Check sheet for the drawn part. Datum: minimum x, y, z corner. Units: mm. A direction names the side the tool comes from. Round coordinates to 2 decimals unless told otherwise and drop trailing zeros. Write each loop counter-clockwise with the first axis right and the second up, starting at its lowest first coordinate (ties: lowest second). Pieces come first, ordered by that corner, then holes. Notation, with made-up numbers: M 21.25,51 L 47.25,51 A10 ccw 47.25,64 Z; hole C 22.25,2.5 d2. An arc over 180 degrees is marked long. Answer in a Markdown table with one row per item. Add a question column.
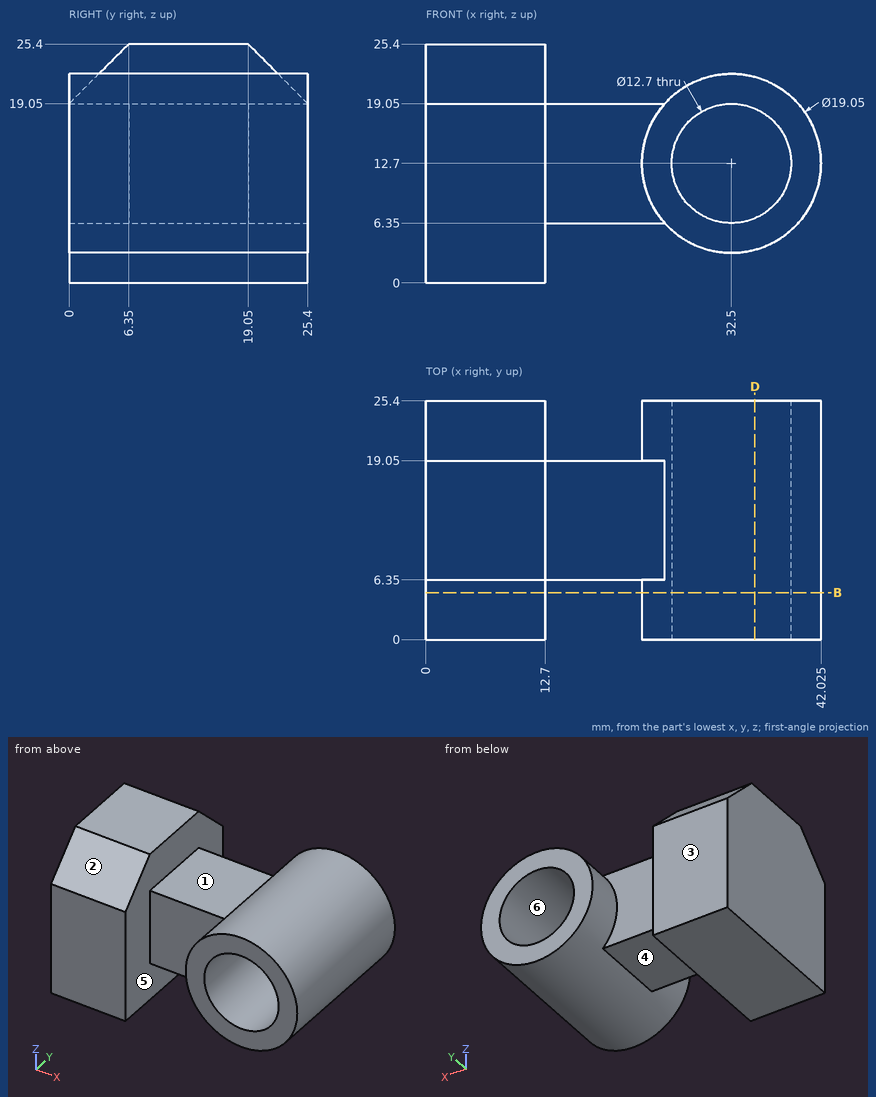
Item 1: Scan lines: probe 1 along X at (y, z) = (22.5, 9) (1 decimal); probe 2 along X at (y, z) = (21.25, 10.25) (1 decimal); probe 3 along Z at (x, y) = (36, 21.75). Record each from-to range of solid material in increasing order. Write a range as from..to.
Item 2: Section check B-B, the plane y = 5. Give the number of separate pieces and of enclosed holes in the cut face, and give its area (3 significant figures).
Item 3: Gauge pin test, flat ends, axial feed: pin 1 Ø7.5 at (y, z) = (7, 14.5) entering from +X (1 decimal); pin 2 Ø5 at (x, y) = (27, 13.5) entering from +Z; pin 3 Ø10 at (x, y) = (21.5, 12) entering from +Z; pin 4 Ø3 at (y, z) = (14.5, 17.5) entering from +X (1 decimal). Record the tip position at first contact, or that the pin passes through.
Item 4: Mould release check, pull along Z, two halves, no side actions. Record for the marked faces 4, 5 and 6: +Z half, -Z half, draft (parallel to the pull), parting line (faces both ways), or undercut.
Item 5: Section check D-D, the plane x = 35. Record the boundary of the cut face in (y, z).
Item 6: Access from +Z, -Z, +X, -X, +Y, -Y to the whole of each face (thin tool, end or side, straight path). Record for the marked faces 1, 2 and 3.
Result sheet:
| question | item | result |
|---|---|---|
| 1 | probe 1 | x = 0..12.7, 23.7..27.3, 37.7..41.3 |
| 1 | probe 2 | x = 0..12.7, 23.3..26.6, 38.4..41.7 |
| 1 | probe 3 | z = 3.84..7.4, 18..21.56 |
| 2 | separate pieces | 2 |
| 2 | enclosed holes | 1 |
| 2 | area | 464 mm^2 |
| 3 | pin 1 | stops at x = 42 |
| 3 | pin 2 | stops at z = 21.74 |
| 3 | pin 3 | stops at z = 20.1 |
| 3 | pin 4 | stops at x = 41.4 |
| 4 | face 4 | -Z half |
| 4 | face 5 | draft |
| 4 | face 6 | undercut |
| 5 | outline | M 0,3.51 L 25.4,3.51 L 25.4,6.86 L 0,6.86 Z; M 0,18.54 L 25.4,18.54 L 25.4,21.89 L 0,21.89 Z |
| 6 | face 1 | +Z, +Y, -Y |
| 6 | face 2 | +Z, -X, -Y |
| 6 | face 3 | +Z, -Z, +X, -X, +Y |
